Check sheet for the modelled part. Datum: model origin and axes. Units: mm. Face numbers are marked on the shaded views. A direction names the side the tool comes from. Round coordinates to 2 decimals unless told otherwise and drop trailing zeros. Write each loop counter-clockwise with the first axis right and the second up, starting at its lowest first coordinate (ties: lowest second). Pieces come first, ordered by that corner, then holes. Notation, with made-up numbers: (66.5, -12) -> (111.5, -12) arc R21 ccw to (111.5, 3) -> close; hole circle Ø3 at (-38.75, 7.25). An arc over 180 degrees is marked (long way). One line per item, written item: value.
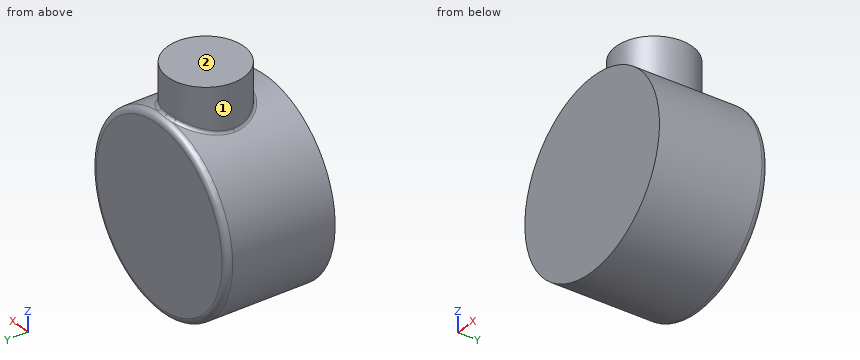
from build123d import *

# Parameters (mm, degrees)
SKETCH1_R           = 60.675
BOSS_EXTRUDE1_DEPTH = 70
SKETCH2_R           = 25
BOSS_EXTRUDE2_DEPTH = 85
FILLET1_R           = 4
FILLET2_R           = 2


with BuildPart() as part:
    # Sketch1 → Boss-Extrude1 (new body)
    with BuildSketch(Plane(origin=(0, 0, 0), x_dir=(1, 0, 0), z_dir=(0, 1, 0))):
        with Locations(Location((0, 0, 0), (0, 0, 270))):
            Circle(SKETCH1_R)
    extrude(amount=BOSS_EXTRUDE1_DEPTH)

    # Sketch2 → Boss-Extrude2 (add)
    with BuildSketch(Plane.XY):
        with Locations(Location((0, 40, 0), (0, 0, 180))):
            Circle(SKETCH2_R)
    extrude(amount=BOSS_EXTRUDE2_DEPTH)

    # Fillet1
    fillet1_edges = [part.edges().sort_by_distance(p)[0] for p in [
        (0, 70, -60.675),
    ]]
    fillet(fillet1_edges, radius=FILLET1_R)

    # Fillet2
    fillet2_edges = [part.edges().sort_by_distance(p)[0] for p in [
        (25, 40, 55.285220674),
    ]]
    fillet(fillet2_edges, radius=FILLET2_R)


solid = part.part
Item 1: Depth check by flat-ended pin: P1, Ø1, axis at y = 40.5, z = 65.5, coming from the +X side; P2, Ø1.5, axis at x = -8.5, z = 38.5, coming from the -Y side; P3, Ø12, axis at x = 46, y = 55, coming from the +Z side; P4, Ø2, axis at x = -46, y = 50.5, coming from the +Z side. Enter the tip coordinate at first touch or a pass-through.
Answer:
P1: stops at x = 25
P2: stops at y = 0
P3: stops at z = 45.62
P4: stops at z = 40.7
Item 2: Tool access check on the marked faces 1 and 2. Record the directions out of +Z, -Z, +X, -X, +Y, -Y that give a thin tool (end or side, any length) a straight path to the whole face; none if there is none.
Answer:
face 1: +Z
face 2: +Z, +X, -X, +Y, -Y
Item 3: Sectioned sample at A-A on y = 11. Enter the section's corners in (x, z) (3 decimals).
Answer:
outline: circle Ø121.35 at (0, 0)
Item 4: Thickness scan on line 1 (Y direction, x = -0.5, z = 69) (3 decimals); line 2 (X direction, y = 60.5, z = 18); line 3 (Z direction, x = -22, y = 35.5). Record the ranges inside material, lowest first.
Answer:
line 1: y = 15.005 to 64.995
line 2: x = -57.94 to 57.94
line 3: z = -56.55 to 85
